Can you work these out from the model? Positions are in its coordinate system, mm. A direction names the side the tool comes from. Coordinates: 2 decimals unless noted, no trailing zeros. Order: outer loops, then holes, each group sorted by start corner. A loop starts at its lowest first (then second) coordinate and runs counter-clockwise, first axis right, second up. Notation, with made-up numbers: (-2.75, 42.5) -> (43.25, 42.5) arc R29 ccw to (43.25, 79.5) -> close; hole circle Ø7 at (58.5, 33.5). An arc over 180 degrees is marked (long way). Answer as CSV lines item,"result".
from build123d import *

# Parameters (mm, degrees)
BOSS_EXTRUDE1_DEPTH = 8
CUT_EXTRUDE1_DEPTH  = 1


with BuildPart() as part:
    # Sketch2 → Boss-Extrude1 (new body)
    with BuildSketch(Plane(origin=(0, 0, 0), x_dir=(1, 0, 0), z_dir=(0, 1, 0))):
        Polygon((3.319764048, 5.75), (-3.319764048, 5.75), (-6.639528096, 0), (-3.319764048, -5.75), (3.319764048, -5.75), (6.639528096, 0), align=None)
    extrude(amount=BOSS_EXTRUDE1_DEPTH)

    # Sketch7 → Cut-Extrude1 (cut)
    with BuildSketch(Plane(origin=(0, 8, 0), x_dir=(1, 0, 0), z_dir=(0, 1, 0))):
        Polygon((-3.921529, 2.029099912), (-3.274393584, 2.029099912), (-3.274393584, -1.470900088), (-3.588496148, -1.470900088), (-3.588496148, 1.670125553), (-4.126957686, 1.670125553), align=None)
        Polygon((-1.229221308, 2.029099912), (-0.582085891, 2.029099912), (-0.582085891, -1.470900088), (-0.896188456, -1.470900088), (-0.896188456, 1.670125553), (-1.434649994, 1.670125553), align=None)
        with BuildLine():
            add(Edge.make_bspline(
                [(1.280093596, -0.932438549), (1.299583808, -0.933596716), (1.33779209, -0.935867166), (1.393031219, -0.95144384), (1.443025878, -0.9791025), (1.487558123, -1.015965279), (1.5242646, -1.060660942), (1.552908952, -1.110256851), (1.568349937, -1.165958443), (1.570603849, -1.204388118), (1.571760262, -1.224105216)],
                knots=[0, 0, 0, 0, 5.8463e-05, 0.000114609, 0.000170453, 0.000228714, 0.000286975, 0.000343156, 0.000399303, 0.000458464, 0.000458464, 0.000458464, 0.000458464], degree=3))
            add(Edge.make_bspline(
                [(1.571760262, -1.224105216), (1.570564662, -1.243348546), (1.568206955, -1.281296109), (1.552944346, -1.336577572), (1.524046296, -1.386204476), (1.487811303, -1.431506615), (1.44301487, -1.468447485), (1.392913023, -1.49587083), (1.337921765, -1.51256281), (1.299605442, -1.514689107), (1.280093596, -1.515771883)],
                knots=[0, 0, 0, 0, 5.7765e-05, 0.000113912, 0.000170093, 0.000228896, 0.000287156, 0.000343, 0.000399343, 0.000457806, 0.000457806, 0.000457806, 0.000457806], degree=3))
            add(Edge.make_bspline(
                [(1.280093596, -1.515771883), (1.26056769, -1.514728285), (1.222448007, -1.51269091), (1.167662013, -1.495528104), (1.117255045, -1.468704644), (1.072467333, -1.431437734), (1.035928861, -1.386437591), (1.008303478, -1.336235794), (0.99171333, -1.281454357), (0.989531457, -1.243379714), (0.988426929, -1.224105216)],
                knots=[0, 0, 0, 0, 5.8463e-05, 0.000114135, 0.000170596, 0.000228856, 0.000287659, 0.000343502, 0.000399846, 0.000457611, 0.000457611, 0.000457611, 0.000457611], degree=3))
            add(Edge.make_bspline(
                [(0.988426929, -1.224105216), (0.989489028, -1.204355836), (0.991562647, -1.165797596), (1.008338307, -1.110598489), (1.035714519, -1.060430049), (1.072719914, -1.016033469), (1.11724421, -0.978846167), (1.167540415, -0.951781374), (1.222579955, -0.935740961), (1.260589894, -0.933558445), (1.280093596, -0.932438549)],
                knots=[0, 0, 0, 0, 5.9161e-05, 0.000115504, 0.000171348, 0.000229609, 0.000287869, 0.00034433, 0.000399803, 0.000458266, 0.000458266, 0.000458266, 0.000458266], degree=3))
        make_face()
        with BuildLine():
            Line((4.21919616, 2.029099912), (4.21919616, 1.670125553))
            Line((4.21919616, 1.670125553), (3.028691352, 1.670125553))
            Line((3.028691352, 1.670125553), (2.840089589, 0.749552637))
            add(Edge.make_bspline(
                [(2.840089589, 0.749552637), (2.877145464, 0.759782909), (2.94893536, 0.779602442), (3.054895221, 0.801608213), (3.155487424, 0.814873657), (3.220762794, 0.816684967), (3.252349205, 0.817561451)],
                knots=[0, 0, 0, 0, 0.000115302, 0.000223379, 0.000324431, 0.000419176, 0.000419176, 0.000419176, 0.000419176], degree=3))
            add(Edge.make_bspline(
                [(3.252349205, 0.817561451), (3.291432944, 0.816715515), (3.368281342, 0.815052194), (3.480720289, 0.799080345), (3.588053182, 0.77394043), (3.690055552, 0.738819908), (3.786916103, 0.693910175), (3.877743664, 0.637810235), (3.963901577, 0.572276904), (4.043844171, 0.496931892), (4.116368479, 0.414010275), (4.180134469, 0.324852404), (4.234297059, 0.230324742), (4.277857814, 0.129524133), (4.312642149, 0.02356498), (4.335794143, -0.088667603), (4.351210852, -0.206115723), (4.352933239, -0.286420293), (4.353811544, -0.32737044)],
                knots=[0, 0, 0, 0, 0.00011719, 0.000230425, 0.000339944, 0.000447481, 0.000553499, 0.000659556, 0.000767111, 0.000877722, 0.000988528, 0.001097091, 0.001206056, 0.001314692, 0.001425996, 0.001539995, 0.001658004, 0.001780798, 0.001780798, 0.001780798, 0.001780798], degree=3))
            add(Edge.make_bspline(
                [(4.353811544, -0.32737044), (4.353146469, -0.355892661), (4.351825307, -0.412551648), (4.345106719, -0.496695849), (4.332171003, -0.579058682), (4.314803279, -0.659651074), (4.292260861, -0.738320446), (4.264971807, -0.815291974), (4.231575779, -0.890086581), (4.194944404, -0.963411976), (4.153697926, -1.033610483), (4.107919419, -1.099259469), (4.059553928, -1.161343751), (4.007512542, -1.219197484), (3.951311547, -1.272440502), (3.89163158, -1.321388783), (3.828948861, -1.366870114), (3.762293619, -1.407038309), (3.693151136, -1.444001265), (3.620522919, -1.474324802), (3.546062218, -1.50143533), (3.468697343, -1.523044858), (3.38860353, -1.539977412), (3.305648754, -1.551478013), (3.220268084, -1.55985445), (3.162393072, -1.560378807), (3.1331585, -1.560643677)],
                knots=[0, 0, 0, 0, 8.5583e-05, 0.000170009, 0.000253005, 0.000335518, 0.000417186, 0.000498352, 0.000580291, 0.000662755, 0.000744161, 0.000824288, 0.000902692, 0.000980133, 0.001057498, 0.001134702, 0.00121156, 0.001289599, 0.001368002, 0.001446531, 0.001525481, 0.001605609, 0.001687289, 0.001770875, 0.001856759, 0.001944425, 0.001944425, 0.001944425, 0.001944425], degree=3))
            add(Edge.make_bspline(
                [(3.1331585, -1.560643677), (3.098284319, -1.559952839), (3.029673488, -1.558593697), (2.929152921, -1.544375212), (2.832438315, -1.524011296), (2.740308214, -1.493375026), (2.651936951, -1.454987731), (2.568514233, -1.40647156), (2.487908457, -1.351492456), (2.41339642, -1.286612103), (2.344240307, -1.215696421), (2.282333798, -1.13873878), (2.227200221, -1.057009338), (2.179722474, -0.970111184), (2.139224453, -0.878272653), (2.107409464, -0.781149652), (2.081731109, -0.679249648), (2.070867689, -0.609096137), (2.065350006, -0.57346419)],
                knots=[0, 0, 0, 0, 0.000104552, 0.000205693, 0.000304023, 0.000400691, 0.00049644, 0.000592535, 0.000689779, 0.000788716, 0.000888377, 0.000986596, 0.001084603, 0.001183757, 0.001283279, 0.001385267, 0.001490017, 0.001598135, 0.001598135, 0.001598135, 0.001598135], degree=3))
            Line((2.065350006, -0.57346419), (2.37945257, -0.57346419))
            add(Edge.make_bspline(
                [(2.37945257, -0.57346419), (2.387181128, -0.606840643), (2.402035844, -0.670992038), (2.434641593, -0.761123379), (2.474507468, -0.841442603), (2.521911817, -0.913012186), (2.578461847, -0.975421183), (2.642991276, -1.031038245), (2.715338999, -1.081213374), (2.795732229, -1.123036142), (2.880545308, -1.158704895), (2.969312518, -1.18245659), (3.059616865, -1.199157483), (3.120695235, -1.200829244), (3.151387666, -1.201669318)],
                knots=[0, 0, 0, 0, 0.000102709, 0.000197412, 0.000286774, 0.000371169, 0.000454082, 0.000538572, 0.000626283, 0.000717552, 0.000809994, 0.00090168, 0.00099274, 0.001084718, 0.001084718, 0.001084718, 0.001084718], degree=3))
            add(Edge.make_bspline(
                [(3.151387666, -1.201669318), (3.181346111, -1.20084854), (3.240334533, -1.199232422), (3.32714592, -1.18679341), (3.410958794, -1.167635839), (3.490946151, -1.138965984), (3.56850769, -1.104121265), (3.641681461, -1.059406189), (3.712584338, -1.007946171), (3.779012471, -0.948989541), (3.83985192, -0.884019846), (3.893608042, -0.814542453), (3.938384955, -0.740425606), (3.976119064, -0.662952454), (4.004772363, -0.581273896), (4.025213344, -0.495772721), (4.037216403, -0.406237741), (4.038867583, -0.345168431), (4.03970898, -0.314049126)],
                knots=[0, 0, 0, 0, 8.9842e-05, 0.0001769, 0.000262612, 0.000347317, 0.000431396, 0.000517249, 0.000604055, 0.000693954, 0.000783242, 0.000870748, 0.000956963, 0.001042571, 0.001128832, 0.00121607, 0.001305907, 0.001399251, 0.001399251, 0.001399251, 0.001399251], degree=3))
            add(Edge.make_bspline(
                [(4.03970898, -0.314049126), (4.039050501, -0.285973374), (4.037761621, -0.231019085), (4.027231051, -0.150619879), (4.008914078, -0.074546837), (3.983490198, -0.002432603), (3.951210691, 0.06579084), (3.911764378, 0.1301939), (3.86441098, 0.189927733), (3.810319092, 0.245020287), (3.751061051, 0.295865162), (3.685617308, 0.339209248), (3.615357382, 0.375673166), (3.541127782, 0.407141164), (3.461162883, 0.429741909), (3.377046251, 0.446709795), (3.287869543, 0.456525158), (3.226898855, 0.457887046), (3.195558339, 0.458587092)],
                knots=[0, 0, 0, 0, 8.4208e-05, 0.000164824, 0.000242709, 0.000318547, 0.000393815, 0.000468731, 0.000544614, 0.00062196, 0.000700062, 0.000778428, 0.000856831, 0.000937299, 0.001019835, 0.001105635, 0.00119452, 0.001288536, 0.001288536, 0.001288536, 0.001288536], degree=3))
            add(Edge.make_bspline(
                [(3.195558339, 0.458587092), (3.168429411, 0.458006501), (3.112415055, 0.456807727), (3.026492228, 0.44798123), (2.936200506, 0.433741936), (2.84188601, 0.414155689), (2.743265502, 0.388524612), (2.640547101, 0.357810111), (2.533514835, 0.321088112), (2.46139711, 0.293355899), (2.424324365, 0.279099912)],
                knots=[0, 0, 0, 0, 8.1378e-05, 0.000168026, 0.000258858, 0.000355524, 0.000456875, 0.000564457, 0.000677092, 0.000796243, 0.000796243, 0.000796243, 0.000796243], degree=3))
            Line((2.424324365, 0.279099912), (2.783298724, 2.029099912))
            Line((2.783298724, 2.029099912), (4.21919616, 2.029099912))
        make_face()
    extrude(amount=-CUT_EXTRUDE1_DEPTH, mode=Mode.SUBTRACT)


solid = part.part
Q1. We'd pull the mould along Z, two halves only. Please class faces 3 (the flat face through (4.956, 3.944, 2.915)), 4 (the flat face through (-4.956, 3.944, -2.915)), 5 (the flat face through (-3.274, 7.5, -0.3)): pulls with the +Z half, pulls with the -Z half, needs draft (parallel to the pull), parting line crosses it, or undercut.
Solution:
face 3,"pulls with the +Z half"
face 4,"pulls with the -Z half"
face 5,"undercut"
Q2. Imagine slicing it at B-B (x = -3.75). List the corners of the cut face in (y, z) for me, and give its area (3 significant figures).
Solution:
outline,"(0, -5) -> (8, -5) -> (8, -2.03) -> (7, -2.03) -> (7, -1.67) -> (8, -1.67) -> (8, 5) -> (0, 5) -> close"
area,"79.7 mm2"
Q3. Imagine slicing it at D-D (z = 3.25). List the corners of the cut face in (x, y) for me.
Solution:
outline,"(-4.76, 0) -> (4.76, 0) -> (4.76, 8) -> (-4.76, 8) -> close"
Q4. For P1, Ø0.7, axis at x = -3.5, z = -0.5, coming from the +Y side; P2, Ø1, axis at x = 4, y = 1.5, coming from the +Z side; P3, Ø2, axis at y = 1, z = 2.5, coming from the -X side; P4, Ø1.5, axis at y = 4.5, z = -3, coming from the -X side, each with a flat end and sliding along its axis, tell me the tip position at first contact or that it passes through.
Solution:
P1,"y = 8"
P2,"z = 5.44"
P3,"x = -5.77"
P4,"x = -5.34"
Q5. Imagine slicing it at C-C (z = 5.25). List the corners of the cut face in (x, y) for me, and give its area (3 significant figures).
Solution:
outline,"(-3.61, 0) -> (3.61, 0) -> (3.61, 8) -> (-3.61, 8) -> close"
area,"57.7 mm2"
Q6. Imagine slicing it at A-A (y = 1.5). List the corners of the cut face in (x, z) for me.
Solution:
outline,"(-6.64, 0) -> (-3.32, -5.75) -> (3.32, -5.75) -> (6.64, 0) -> (3.32, 5.75) -> (-3.32, 5.75) -> close"
Q7. Which directions (+Z, -Z, +X, -X, +Y, -Y) give clear straight access to the entire face, cutting with the end or side of a thin tool? Please do faces 1 (the flat face through (-3.588, 7.5, -0.1)), 2 (the flat face through (0, 8, 0)).
Solution:
face 1,"+Y"
face 2,"+Z, -Z, +X, -X, +Y"
Q8. If I drill on line 1 (X direction, y = 5.5, z = -0.75); line 2 (X direction, y = 3.5, z = 3); line 3 (Z direction, x = -3.5, y = 1.5), over which ranges is the centre line in solid material (lowest first)?
Solution:
line 1,"-6.21 to 6.21"
line 2,"-4.91 to 4.91"
line 3,"-5.44 to 5.44"
